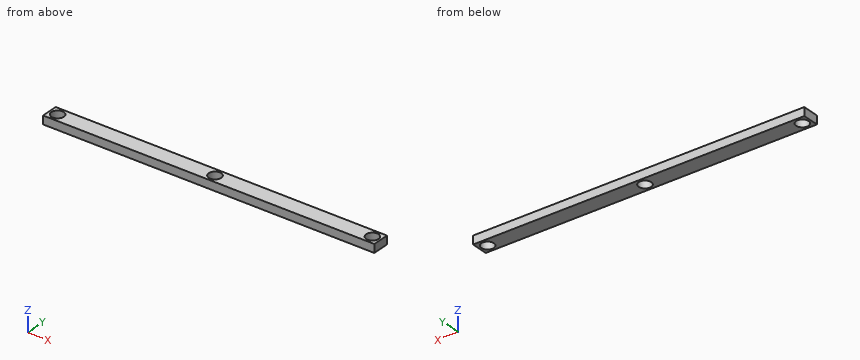
from build123d import *

# Parameters (mm, degrees)
SKETCH1_W           = 40
SKETCH1_H           = 10
BOSS_EXTRUDE1_DEPTH = 2
SKETCH4_W           = 40
SKETCH4_H           = 9
CUT_EXTRUDE2_DEPTH  = 2
SKETCH5_R           = 0.75
CUT_EXTRUDE3_DEPTH  = 41.062451248


with BuildPart() as part:
    # Sketch1 → Boss-Extrude1 (new body)
    with BuildSketch(Plane(origin=(0, 0, 0), x_dir=(1, 0, 0), z_dir=(0, 1, 0))):
        with Locations((20, 5)):
            Rectangle(SKETCH1_W, SKETCH1_H)
    extrude(amount=BOSS_EXTRUDE1_DEPTH)

    # Sketch4 → Cut-Extrude2 (cut)
    with BuildSketch(Plane(origin=(0, 2, 0), x_dir=(1, 0, 0), z_dir=(0, 1, 0))):
        with Locations((20, 5.5)):
            Rectangle(SKETCH4_W, SKETCH4_H)
    extrude(amount=-CUT_EXTRUDE2_DEPTH, mode=Mode.SUBTRACT)

    # Sketch5 → Cut-Extrude3 (cut, through all)
    with BuildSketch(Plane.XY):
        with Locations((20, 1)):
            Circle(SKETCH5_R)
        with Locations((1, 1)):
            Circle(SKETCH5_R)
        with Locations((39, 1)):
            Circle(SKETCH5_R)
    extrude(amount=-CUT_EXTRUDE3_DEPTH, mode=Mode.SUBTRACT)


solid = part.part
Work out the finished part from the listing and answer in its coordinate system (mm). Coordinates: 2 decimals unless noted, no trailing zeros. Write each loop counter-clockwise with the first axis right and the second up, starting at its lowest first coordinate (ties: lowest second). Pieces come first, ordered by that corner, then holes. Notation, with made-up numbers: (66.5, 70) - (87.5, 70) arc R21 cw to (87.5, 79) - close; hole circle Ø8 at (0, -1). An arc over 180 degrees is marked (long way). One line per question, with ' | ' between items.
1) Find section C-C, the plane x = 1. Determine the outline of the cut face in (y, z).
Checks:
outline: (0, -1) - (0.25, -1) - (0.25, 0) - (0, 0) - close; (1.75, -1) - (2, -1) - (2, 0) - (1.75, 0) - close
2) A flat-ended cylindrical pin translates along its axis: P1, Ø1.2, axis at x = 1, y = 1, coming from the -Z side. Find the tip coordinate at first contact, or state that the pin passes through.
Checks:
P1: through
3) Consider probe 1 along X at (y, z) = (0.95, -0.55); probe 2 along X at (y, z) = (1.5, -0.05); probe 3 along Y at (x, z) = (20, -0.45). Determine where each line is inside the solid, lowest interval first. Write a range as [from, to].
Checks:
probe 1: [0, 0.25], [1.75, 19.25], [20.75, 38.25], [39.75, 40] | probe 2: [0, 0.44], [1.56, 19.44], [20.56, 38.44], [39.56, 40] | probe 3: [0, 0.25], [1.75, 2]
4) Find section A-A, the plane z = -0.35. Determine the outline of the cut face in (x, y).
Checks:
outline: (0, 0) - (40, 0) - (40, 2) - (0, 2) - close; hole circle Ø1.5 at (1, 1); hole circle Ø1.5 at (20, 1); hole circle Ø1.5 at (39, 1)
5) Find section B-B, the plane y = 1. Determine the outline of the cut face in (x, z), and give its area (3 significant figures).
Checks:
outline: (0, -1) - (0.25, -1) - (0.25, 0) - (0, 0) - close; (1.75, -1) - (19.25, -1) - (19.25, 0) - (1.75, 0) - close; (20.75, -1) - (38.25, -1) - (38.25, 0) - (20.75, 0) - close; (39.75, -1) - (40, -1) - (40, 0) - (39.75, 0) - close | area: 35.5 mm2
